Can you work these out from the model? Positions are in its coordinate system, mm. A direction names the side the tool comes from. Give positions to 0.01 mm unless a question says otherwise; leave off trailing zeros. Loops run counter-clockwise (first coordinate to the right, second up) from the corner with the lowest first, then second, coordinate; pieces in that order, holes last. Notation, with made-up numbers: (-18.5, 88.25) -> (28.5, 88.25) arc R22 cw to (28.5, 118.25) -> close; hole circle Ø6 at (76.5, -24.5). An arc over 180 degrees is marked (long way). Use CSV: the item, a comma, the result in double quotes.
from build123d import *


with BuildPart() as f1:
    # F0 (on Front) → F1 (revolve)
    with BuildSketch(Plane.XZ):
        with BuildLine():
            ThreePointArc((6, 9.24921), (12.110392, 23.31158), (0, 32.715066))
            Line((0, 32.715066), (0, -7.284934))
            Line((0, -7.284934), (9.5, -7.284934))
            Line((9.5, -7.284934), (9.5, -37.284934))
            Line((9.5, -37.284934), (10.85, -37.284934))
            Line((10.85, -37.284934), (10.85, -17.284934))
            Line((10.85, -17.284934), (10.5, -17.284934))
            Line((10.5, -17.284934), (10.5, -12.284934))
            Line((10.5, -12.284934), (10.85, -12.284934))
            Line((10.85, -12.284934), (10.85, -7.284934))
            Line((10.85, -7.284934), (12.5, -7.284934))
            Line((12.5, -7.284934), (12.5, -5.284934))
            Line((12.5, -5.284934), (6, 1.715066))
            Line((6, 1.715066), (6, 9.24921))
        make_face()
    revolve(axis=Axis((0, 0, 12.715066), (0, 0, -1)))


solid = f1.part
(1) We'd pull the mould along Y, two halves only. Please class faces 4 (the face through (0, 0, -7.285)), 5 (the face through (0, 10, -37.285)), 6 (the face through (-8, -7.33, -27.14)): released by +Y, released by -Y, zero draft, split by the parting line, or undercut.
Answer sheet:
face 4,"undercut"
face 5,"zero draft"
face 6,"split by the parting line"
(2) Which directions (+Z, -Z, +X, -X, +Y, -Y) give clear straight access to the entire face, cutting with the end or side of a thin tool? Please do faces 1 (the face through (11.923, -3.755, -6.271)), 2 (the face through (4.38, 8.43, -22.49)), 3 (the face through (10, -3.2, -14.7)).
Answer sheet:
face 1,"+Z, -Z"
face 2,"-Z"
face 3,"none"
(3) If I drill on L1, parallel to Y at x = 0, z = -28.5; L2, parallel to Y at x = 0, z = -15, over which ranges is the centre line in solid material (lowest first)? Write a range as from..to.
Answer sheet:
L1,"y = -10.85..-9.5, 9.5..10.85"
L2,"y = -10.5..-9.5, 9.5..10.5"
(4) If we section it at A-A, the plane z = 5: Write out the boundary of the cut face in (x, y), then the cut area to 3 significant figures.
Answer sheet:
outline,"circle Ø12 at (0, 0)"
area,"113 mm2"
(5) Will these pins go through, and if not, where does the flat tip stop? pin 1 Ø1.5 at (x, y) = (1.5, 3.5) entering from +Z; pin 2 Ø2 at (x, z) = (6.5, -30) entering from -Y; pin 3 Ø6.5 at (x, y) = (-4.5, -1.5) entering from -Z.
Answer sheet:
pin 1,"stops at z = 32.34"
pin 2,"stops at y = -9.35"
pin 3,"stops at z = -7.28"
